```python
from build123d import *

# Parameters (mm, degrees)
CROQUIS1_W              = 50
CROQUIS1_H              = 56
SALIENTE_EXTRUIR1_DEPTH = 47
SALIENTE_EXTRUIR2_DEPTH = 56
CROQUIS3_W              = 44
CROQUIS3_H              = 69.477636763
CORTAR_EXTRUIR1_DEPTH   = 93.021736563
CROQUIS4_R              = 4
CROQUIS4_R_2            = 1.6
CORTAR_EXTRUIR2_DEPTH   = 95.578010129
CROQUIS5_R              = 1.55
CORTAR_EXTRUIR3_DEPTH   = 76.927597091


with BuildPart() as part:
    # Croquis1 → Saliente-Extruir1 (new body)
    with BuildSketch(Plane(origin=(0, 0, 0), x_dir=(1, 0, 0), z_dir=(0, 1, 0))):
        Rectangle(CROQUIS1_W, CROQUIS1_H)
    extrude(amount=SALIENTE_EXTRUIR1_DEPTH)

    # Croquis2 → Saliente-Extruir2 (add)
    with BuildSketch(Plane.XY.offset(28)):
        with BuildLine():
            Line((-25, 47), (25, 47))
            ThreePointArc((25, 47), (0, 72), (-25, 47))
        make_face()
    extrude(amount=-SALIENTE_EXTRUIR2_DEPTH)

    # Croquis3 → Cortar-Extruir1 (cut, through all)
    with BuildSketch(Plane.ZY.offset(25)):
        with Locations((0, 40.738818382)):
            Rectangle(CROQUIS3_W, CROQUIS3_H)
    extrude(amount=-CORTAR_EXTRUIR1_DEPTH, mode=Mode.SUBTRACT)

    # Croquis4 → Cortar-Extruir2 (cut, through all)
    with BuildSketch(Plane.XY.offset(28)):
        with Locations((0, 57)):
            Circle(CROQUIS4_R)
        with Locations((-12, 57)):
            Circle(CROQUIS4_R_2)
    extrude(amount=-CORTAR_EXTRUIR2_DEPTH, mode=Mode.SUBTRACT)

    # Croquis5 → Cortar-Extruir3 (cut, through all)
    with BuildSketch(Plane(origin=(0, 6, 0), x_dir=(1, 0, 0), z_dir=(0, 1, 0))):
        with Locations(Location((13, -14.15, 0), (0, 0, 270))):
            Circle(CROQUIS5_R)
        with Locations(Location((13, 14.15, 0), (0, 0, 270))):
            Circle(CROQUIS5_R)
        with Locations(Location((-12, 0, 0), (0, 0, 270))):
            Circle(CROQUIS5_R)
    extrude(amount=-CORTAR_EXTRUIR3_DEPTH, mode=Mode.SUBTRACT)


solid = part.part
```
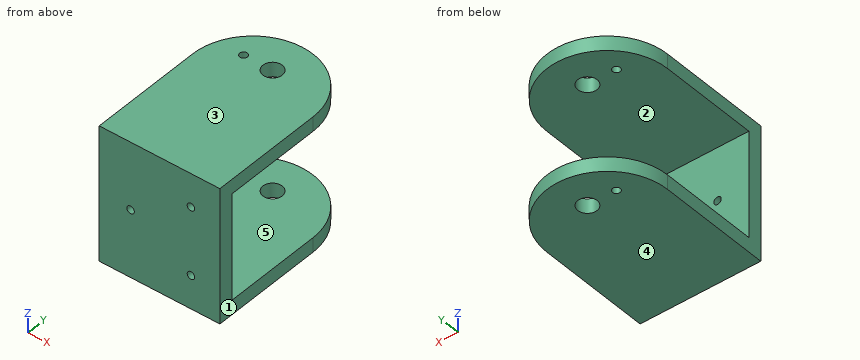
Input: part model. Units: mm. Frame: model coordinates. Face numbers are marked on the shaded views. A direction names the side the tool comes from. Round coordinates to 2 decimals unless told otherwise and drop trailing zeros. Loops run counter-clockwise (first coordinate to the right, second up) from the corner with the lowest first, then second, coordinate; pieces in that order, holes last. Notation, with made-up numbers: M 26.5,-21.75 L 59.5,-21.75 A21 ccw 59.5,16.25 Z; hole C -37.75,68.25 d6. An arc over 180 degrees is marked long. Answer in a Markdown table with one row per item. Add a question column.
1. Ray query, probe 1 along Z at (x, y) = (14, 34); probe 2 along Y at (x, z) = (0, 24.4); probe 3 along Y at (x, z) = (-4, 16.5). Return the intervals inside material, ascending.
2. Section C-C (z = 0). Output: boundary loops of the cut face in (x, y).
3. Contact query for a flat-ended pin moving along its axis: pin 1 (6 mm diameter, centred on x = -17.5, z = -11.5, fed in from +Y). Output: stop coordinate, or through.
4. Section D-D (x = -12). Output: boundary loops of the cut face in (y, z).
5. Set-up query: the marked faces 4 and 5. Return all of +Z, -Z, +X, -X, +Y, -Y with unobstructed straight access to the full face (end or side cutting, diameter ignored); none if empty.
6. Mould query, pull axis Z, two halves, no side actions, for the marked faces 1, 2 and 3. Classes: released by +Z, released by -Z, zero draft, split by the parting line, or undercut.
7. Section A-A (x = 0). Output: boundary loops of the cut face in (y, z), and give its area (3 significant figures).
8. Section B-B (y = 34). Output: boundary loops of the cut face in (x, z).
Values follow:
| question | item | result |
|---|---|---|
| 1 | probe 1 | -28 to -22, 22 to 28 |
| 1 | probe 2 | 0 to 53, 61 to 72 |
| 1 | probe 3 | 0 to 6 |
| 2 | outline | M -25,0 L -13.55,0 L -13.55,6 L -25,6 Z; M -10.45,0 L 25,0 L 25,6 L -10.45,6 Z |
| 3 | pin 1 | y = 6 |
| 4 | outline | M 0,-28 L 55.4,-28 L 55.4,-22 L 6,-22 L 6,-1.55 L 0,-1.55 Z; M 0,1.55 L 6,1.55 L 6,22 L 55.4,22 L 55.4,28 L 0,28 Z; M 58.6,-28 L 68.93,-28 L 68.93,-22 L 58.6,-22 Z; M 58.6,22 L 68.93,22 L 68.93,28 L 58.6,28 Z |
| 5 | face 4 | -Z, +X, -X, +Y, -Y |
| 5 | face 5 | +X, -X, +Y |
| 6 | face 1 | zero draft |
| 6 | face 2 | undercut |
| 6 | face 3 | released by +Z |
| 7 | outline | M 0,-28 L 53,-28 L 53,-22 L 6,-22 L 6,22 L 53,22 L 53,28 L 0,28 Z; M 61,-28 L 72,-28 L 72,-22 L 61,-22 Z; M 61,22 L 72,22 L 72,28 L 61,28 Z |
| 7 | area | 1,030 mm^2 |
| 8 | outline | M -25,-28 L 25,-28 L 25,-22 L -25,-22 Z; M -25,22 L 25,22 L 25,28 L -25,28 Z |
